from build123d import *

# Parameters (mm, degrees)
SKETCH9_W           = 28.5
SKETCH9_H           = 42.5
BOSS_EXTRUDE2_DEPTH = 20
SHELL1_T            = 2
SKETCH13_R          = 4
CUT_EXTRUDE3_DEPTH  = 20
CUT_EXTRUDE4_DEPTH  = 45
SKETCH16_R          = 5
CUT_EXTRUDE5_DEPTH  = 9
CUT_EXTRUDE6_DEPTH  = 9
SKETCH18_W          = 10.869116721
SKETCH18_H          = 10.889459445
CUT_EXTRUDE7_DEPTH  = 1
SKETCH19_W          = 32.5
SKETCH19_H          = 46.5
SKETCH19_W_2        = 28.5
SKETCH19_H_2        = 42.5
BOSS_EXTRUDE3_DEPTH = 16
SKETCH21_R          = 1.5
BOSS_EXTRUDE4_DEPTH = 23.937925
SKETCH22_R          = 1.499227017
BOSS_EXTRUDE5_DEPTH = 23.937925
SKETCH24_W          = 8
SKETCH24_H          = 10
CUT_EXTRUDE9_DEPTH  = 25
CUT_EXTRUDE11_DEPTH = 5
CUT_EXTRUDE12_DEPTH = 5
FILLET1_R           = 2


with BuildPart() as part:
    # Sketch9 → Boss-Extrude2 (new body)
    with BuildSketch(Plane(origin=(0, 0, 0), x_dir=(0, 0, -1), z_dir=(1, 0, 0))):
        with Locations((-0.252212389, -5.10840708)):
            Rectangle(SKETCH9_W, SKETCH9_H)
    extrude(amount=BOSS_EXTRUDE2_DEPTH)

    # Shell1
    shell1_openings = [part.faces().sort_by_distance(p)[0] for p in [
        (20, -5.10840708, 0.252212389),
    ]]
    offset(amount=SHELL1_T, openings=shell1_openings, kind=Kind.INTERSECTION)

    # Sketch13 → Cut-Extrude3 (cut)
    with BuildSketch(Plane.ZY.offset(2)):
        with Locations((0.252212389, 6.14159292)):
            Circle(SKETCH13_R)
        Polygon((13.97143347, -17.263089004), (14.536325863, -14.432147479), (12.367104782, -12.527465555), (9.632991308, -13.453725155), (9.068098916, -16.28466668), (11.237319997, -18.189348605), align=None)
    extrude(amount=-CUT_EXTRUDE3_DEPTH, mode=Mode.SUBTRACT)

    # Sketch14 → Cut-Extrude4 (cut)
    with BuildSketch(Plane.XY.offset(16.502212389)):
        Polygon((5.937924746, 21.010526575), (5.937924746, -38.52738051), (34.577859994, -38.52738051), (26.806020853, 26.17065701), align=None)
    extrude(amount=-CUT_EXTRUDE4_DEPTH, mode=Mode.SUBTRACT)

    # Sketch16 → Cut-Extrude5 (cut)
    with BuildSketch(Plane.ZY.offset(2)):
        with Locations((0.252212389, 6.14159292)):
            Circle(SKETCH16_R)
    extrude(amount=-CUT_EXTRUDE5_DEPTH, mode=Mode.SUBTRACT)

    # Sketch17 → Cut-Extrude6 (cut)
    with BuildSketch(Plane.ZY.offset(2)):
        Polygon((13.82530443, -17.774965015), (15.201707449, -14.192469286), (12.787376648, -11.209221442), (8.996642829, -11.808469327), (7.62023981, -15.390965055), (10.034570611, -18.3742129), align=None)
    extrude(amount=-CUT_EXTRUDE6_DEPTH, mode=Mode.SUBTRACT)

    # Sketch18 → Cut-Extrude7 (cut)
    with BuildSketch(Plane(origin=(0, 0, 0), x_dir=(0, 0, -1), z_dir=(1, 0, 0))):
        with Locations((-0.252212389, 6.141592921)):
            Rectangle(SKETCH18_W, SKETCH18_H)
    extrude(amount=-CUT_EXTRUDE7_DEPTH, mode=Mode.SUBTRACT)

    # Sketch19 → Boss-Extrude3 (add)
    with BuildSketch(Plane(origin=(5.937924746, 0, 0), x_dir=(0, 0, -1), z_dir=(1, 0, 0))):
        with Locations((-0.252212389, -5.10840708)):
            Rectangle(SKETCH19_W, SKETCH19_H)
        with Locations((-0.252212389, -5.10840708)):
            Rectangle(SKETCH19_W_2, SKETCH19_H_2, mode=Mode.SUBTRACT)
    extrude(amount=BOSS_EXTRUDE3_DEPTH)

    # Sketch21 → Boss-Extrude4 (add)
    with BuildSketch(Plane(origin=(21.937924746, 0, 0), x_dir=(0, 0, -1), z_dir=(1, 0, 0))):
        with Locations((-14.502212389, -26.35840708)):
            Circle(SKETCH21_R)
    extrude(amount=-BOSS_EXTRUDE4_DEPTH)

    # Sketch22 → Boss-Extrude5 (add)
    with BuildSketch(Plane(origin=(21.937924746, 0, 0), x_dir=(0, 0, -1), z_dir=(1, 0, 0))):
        with Locations((13.997787611, 16.14159292)):
            Circle(SKETCH22_R)
    extrude(amount=-BOSS_EXTRUDE5_DEPTH)

    # Sketch24 → Cut-Extrude9 (cut)
    with BuildSketch(Plane.XZ.offset(28.35840708)):
        with Locations((11.762438337, -0.163014209)):
            Rectangle(SKETCH24_W, SKETCH24_H)
    extrude(amount=-CUT_EXTRUDE9_DEPTH, mode=Mode.SUBTRACT)

    # Sketch25 → Cut-Extrude11 (cut)
    with BuildSketch(Plane(origin=(21.937924746, 0, 0), x_dir=(0, 0, -1), z_dir=(1, 0, 0))):
        Polygon((15.997787611, 18.14159292), (15.997787611, -28.35840708), (14.997787611, -28.35840708), (14.997787611, -27.35840708), (14.997787611, 17.14159292), (-14.502212389, 17.14159292), (-16.502212389, 17.14159292), (-16.502212389, 18.14159292), align=None)
    extrude(amount=-CUT_EXTRUDE11_DEPTH, mode=Mode.SUBTRACT)

    # Sketch26 → Cut-Extrude12 (cut)
    with BuildSketch(Plane(origin=(21.937924746, 0, 0), x_dir=(0, 0, -1), z_dir=(1, 0, 0))):
        Polygon((14.997787611, -28.35840708), (14.997787611, -27.35840708), (-15.502212389, -27.35840708), (-15.502212389, 17.14159292), (-16.502212389, 17.14159292), (-16.502212389, -28.35840708), align=None)
    extrude(amount=-CUT_EXTRUDE12_DEPTH, mode=Mode.SUBTRACT)

    # Fillet1
    fillet1_edges = [part.edges().sort_by_distance(p)[0] for p in [
        (19.437924746, 17.14159292, -14.997787611),
        (19.437924746, -27.35840708, 15.502212389),
    ]]
    fillet(fillet1_edges, radius=FILLET1_R)


solid = part.part
Design review of the part built by this model. Coordinates are the model's own, in mm. A direction names the side the tool comes from. Round coordinates to 2 decimals unless told otherwise and drop trailing zeros. Write each loop counter-clockwise with the first axis right and the second up, starting at its lowest first coordinate (ties: lowest second). Pieces come first, ordered by that corner, then holes. Notation, with made-up numbers: (-1.5, 9) - (3.5, 9) arc R20 ccw to (3.5, 26) - close; hole circle Ø8 at (30, 1.5). An arc over 180 degrees is marked (long way). Return JSON: item names as keys, results as strings. Group by question number.
Item 1: We need section B-B on x = -0.5. Give the number of separate pieces and of enclosed holes in the cut face, and give its area (3 significant figures).
Item 2: Machinability: for faces 1 (the face through (-1.01, -17.98, 12.53)), 2 (the face through (15.762, -27, 0)), 3 (the face through (11, -6, -13.998)), 4 (the face through (19, -6, -14.998)), 5 (the face through (19.4, -26.76, 14.93)), which of the approach directions +Z, -Z, +X, -X, +Y, -Y give a long, thin tool a straight path to every point of the face, cutting with its end or side? Answer none if there is none.
Item 3: For probe 1 along Y at (x, z) = (19, 9.5); probe 2 along Y at (x, z) = (-0.25, 1.5); probe 3 along Z at (x, y) = (11, 8.5), list the stretches that pass through material, from the lowest coordinate up. Write a range as [from, to].
Item 4: The part is to be moulded in two halves that separate along Z. For faces 6 (the face through (7, -5, 16.502)), 7 (the face through (16.938, -5, -15.5)), 8 (the face through (0, -5, 0)), say which applies: pulls with the +Z half, pulls with the -Z half, needs draft (parallel to the pull), parting line crosses it, or undercut.
Item 5: Insertion check: P1, Ø1.5, axis at x = 18.5, z = -1.5, coming from the +Y side; P2, Ø1.5, axis at x = 20, y = -14, coming from the -Z side; P3, Ø3.5, axis at y = 8, z = -0.5, coming from the +X side; P4, Ø2.5, axis at x = 19, y = -11, coming from the +Z side. Each pin has a flat end and moves straight along its axis. Give the tip position at first contact, or say it passes through.
Item 6: We need section A-A on y = -10. Write out the cut boundary in (x, z).
Item 7: We need section C-C on z = 3. Write out the cut boundary in (x, y).
Item 8: We need section D-D on y = 2. Write out the cut boundary in (x, z).
Model answer:
{
 "1": {"separate pieces": "1", "enclosed holes": "2", "area": "1,350 mm²"},
 "2": {"face 1": "+X, -X", "face 2": "-Y", "face 3": "+X", "face 4": "-Z, +X, +Y, -Y", "face 5": "+Z, +X, -Y"},
 "3": {"probe 1": "y = [-27.36, -26.36], [16.14, 17.14]", "probe 2": "y = [-28.36, 0.7], [11.59, 18.14]", "probe 3": "z = [-16, -14], [14.5, 16.5]"},
 "4": {"face 6": "pulls with the +Z half", "face 7": "needs draft", "face 8": "undercut"},
 "5": {"P1": "stops at y = 17.14", "P2": "stops at z = -15", "P3": "passes through", "P4": "stops at z = 15.5"},
 "6": {"outline": "(-2, -16) - (16.94, -16) - (16.94, -15) - (21.94, -15) - (21.94, -14) - (0, -14) - (0, 14.5) - (21.94, 14.5) - (21.94, 15.5) - (16.94, 15.5) - (16.94, 16.5) - (-2, 16.5) - close"},
 "7": {"outline": "(-2, -28.36) - (7.76, -28.36) - (7.76, -26.36) - (0, -26.36) - (0, 0.7) - (-1, 0.7) - (-1, 1.96) - (-2, 1.96) - close; (-2, 10.32) - (-1, 10.32) - (-1, 11.59) - (0, 11.59) - (0, 16.14) - (21.94, 16.14) - (21.94, 17.14) - (16.94, 17.14) - (16.94, 18.14) - (-2, 18.14) - close; (15.76, -28.36) - (16.94, -28.36) - (16.94, -27.36) - (21.94, -27.36) - (21.94, -26.36) - (15.76, -26.36) - close"},
 "8": {"outline": "(-2, -16) - (16.94, -16) - (16.94, -15) - (21.94, -15) - (21.94, -14) - (0, -14) - (0, -5.18) - (-1, -5.18) - (-1, -2.55) - (-2, -2.55) - close; (-2, 3.05) - (-1, 3.05) - (-1, 5.69) - (0, 5.69) - (0, 14.5) - (21.94, 14.5) - (21.94, 15.5) - (16.94, 15.5) - (16.94, 16.5) - (-2, 16.5) - close"}
}
